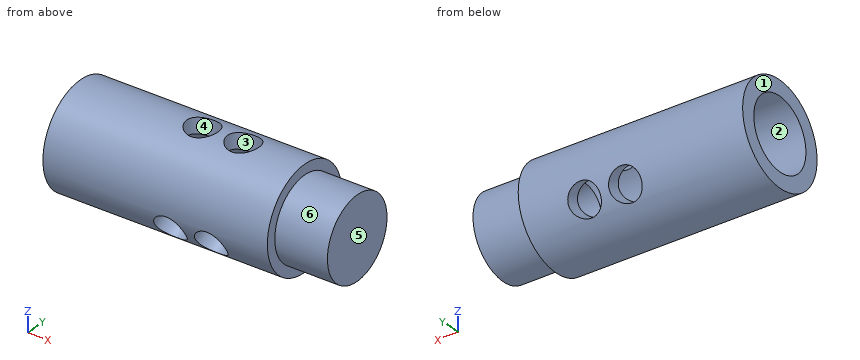
Autodesk Inventor part; units mm, degrees
ref_plane "YZ Plane" through (0, 0, 0) normal (1, 0, 0) x (0, 1, 0)
ref_plane "XZ Plane" through (0, 0, 0) normal (0, 1, 0) x (-1, 0, 0)
ref_plane "XY Plane" through (0, 0, 0) normal (0, 0, 1) x (1, 0, 0)
sketch "Sketch4" plane through (0, 0, 0) normal (0, 0, 1) x (1, 0, 0)
  line L0 (0, 0) -> (0, 5.5562) construction
  line L1 (0, 5.5562) -> (20.1197, 5.5563)
  line L2 (0, 7.9375) -> (26.1937, 7.9375)
  line L3 (26.1937, 7.9375) -> (26.1937, 6.35)
  line L4 (26.1937, 5.5563) -> (26.1937, 0) construction
  line L5 (26.1937, 0) -> (0, 0) construction
  line L6 (26.1937, 6.35) -> (34.3852, 6.35)
  line L7 (26.1937, 0) -> (31.75, 0) construction
  line L8 (34.3852, 0) -> (34.3852, 6.35)
  line L9 (16.6687, 7.9375) -> (16.6687, 0) construction
  circle A0 centre (16.6687, 7.5565) radius 2.3813 construction
  circle A1 centre (16.6687, 5.4928) radius 2.3813 construction
  circle A2 centre (10.3187, 7.5565) radius 2.3813 construction
  circle A3 centre (10.3187, 5.4928) radius 2.3813 construction
  line L10 (10.3187, 7.9375) -> (10.3187, 0) construction
  line L11 (0, 5.1753) -> (26.1938, 5.1753) construction
  line L12 (8.7312, 5.1753) -> (8.7312, 0) construction
  line L13 (5.5562, 5.1753) -> (5.5562, 0) construction
  line L14 (18.2563, 5.1753) -> (18.2562, 0) construction
  line L15 (21.4313, 5.1753) -> (21.4312, 0) construction
  line L16 (0, 3.1115) -> (26.1937, 3.1115) construction
  line L17 (5.5562, 3.1115) -> (8.7312, 5.1753) construction
  line L18 (18.2563, 5.1753) -> (21.4312, 3.1115) construction
  line L19 (11.9062, 5.1753) -> (11.9062, 0) construction
  line L20 (15.0812, 5.1753) -> (15.0812, 0) construction
  line L21 (11.9062, 5.1753) -> (15.0812, 3.1115) construction
  line L22 (21.4312, 3.3734) -> (29.723, 3.3734)
  line L23 (24.6062, 3.3734) -> (24.6062, 0) construction
  line L24 (21.4312, 3.3734) -> (20.1197, 5.5563)
  line L25 (26.1937, 3.1115) -> (30.9562, 3.1115) construction
  line L26 (30.9562, 3.1115) -> (30.9562, 0) construction
  line L27 (31.75, 3.3734) -> (31.75, 0) construction
  line L28 (31.75, 0) -> (29.723, 3.3734)
  line L29 (0, 7.9375) -> (-1.5875, 7.9375) construction
  line L30 (-1.5875, 7.9375) -> (-1.5875, 3.3734) construction
  line L31 (-1.5875, 3.3734) -> (5.5562, 3.3734) construction
  line L32 (0, 5.5562) -> (0, 7.9375)
  line L33 (0, 7.9375) -> (0, 12.7) construction
  line L34 (20.1197, 5.5563) -> (26.1937, 5.5563) construction
  line L35 (29.723, 3.3734) -> (34.3852, 3.3734) construction
  line L36 (26.1937, 6.35) -> (26.1937, 5.5563) construction
  line L37 (31.75, 0) -> (34.3852, 0)
  line L38 (0, 5.5562) -> (-8.7313, 5.5563)
  line L39 (-8.7313, 5.5563) -> (-8.7313, 7.9375)
  line L40 (-8.7313, 7.9375) -> (0, 7.9375)
  line L41 (-8.7313, 6.35) -> (0, 6.35)
  dimension "d16" = 12.7
  dimension "d17" = 5.5563
  dimension "d18" = 7.9375
  dimension "d19" = 26.1938
  dimension "d20" = 8.1915
  dimension "d21" = 6.35
  dimension "d22" = 9.525
  dimension "d23" = 6.35
  dimension "d24" = 0.381
  dimension "d25" = 0.381
  dimension "d26" = 0.0635
  dimension "d27" = 0.0635
  dimension "d28" = 1.5875
  dimension "d29" = 4.7625
  dimension "d30" = 1.5875
  dimension "d31" = 4.7625
  dimension "d32" = 3.1115
  dimension "d33" = 1.5875
  dimension "d34" = 4.7625
  dimension "d35" = 3.3734
  dimension "d36" = 3.175
  dimension "d37" = 31
  dimension "d38" = 9.525
  dimension "d39" = 9.525
  dimension "d40" = 0.7937
  dimension "d41" = 31
  dimension "d42" = 1.5875
  dimension "d43" = 3.3734
  dimension "d49" = 4.7625
  dimension "d63" = 8.7312
  dimension "d64" = 6.35
revolve "Revolution1" add sketch "Sketch4" angle 360 about axis through (26.1937, 0, 0) along (-1, 0, 0)
sketch "Sketch5" plane through (0, 0, 0) normal (0, 0, 1) x (1, 0, 0)
  line L0 (26.1937, -7.9375) -> (26.1937, 7.9375)
  line L1 (0, 0) -> (26.1937, 0) construction
  circle A0 centre (16.6687, 0) radius 2.4574
  circle A1 centre (10.3187, 0) radius 2.4574
  dimension "d51" = 4.9149
  dimension "d53" = 6.35
  dimension "d54" = 9.525
  dimension "d55" = 4.9149
extrude "Extrusion4" cut sketch "Sketch5" along normal through all
pattern_circular "Circular Pattern2" count 3 over 360 about axis through (-4.3656, 0, 0) along (1, 0, 0) of "Extrusion4"
ref_plane "Work Plane1" through (16.6687, 0, 0) normal (1, 0, 0) x (0, 0, -1)
ref_plane "Work Plane2" through (10.3187, 0, 0) normal (1, 0, 0) x (0, 0, -1)
equation "\"d17\" = d44"
equation "\"d18\" = d45"
equation "\"d24\" = d46"
equation "\"d25\" = d24"
equation "\"d26\" = d47"
equation "\"d27\" = d26"
equation "\"d32\" = d48"
equation "\"d33\" = d28"
equation "\"d34\" = d29"
equation "\"d39\" = d38"
equation "\"d41\" = d37"
equation "\"d43\" = d35"
equation "\"d55\" = d51"
properties part number "Output SHaft"
Can you work these out from the model? Positions are in its coordinate system, mm. Face numbers are marked on the shaded views. A direction names the side the tool comes from. Round coordinates to 2 decimals unless told otherwise and drop trailing zeros. Loops run counter-clockwise (first coordinate to the right, second up) from the corner with the lowest first, then second, coordinate; pieces in that order, holes last. Notation, with made-up numbers: M 4.25,-31 L 23.25,-31 A26 ccw 23.25,-8 Z; hole C 50.5,-10.5 d2. An arc over 180 degrees is marked long. Answer as a JSON object with one key per item and string values. Group by question number.
Q1. On a 3-axis mill with a long thin cutter (end or side, diameter ignored), from which of +Z, -Z, +X, -X, +Y, -Y can I reach the whole of each face in a straight line? I mean the marked faces 1, 2 and 3. Say none if no direction works.
Q2. Imagine slicing it at A-A, the plane x = 28. Please give me the cut outline in (y, z), then the cut area to 3 significant figures.
Q3. Imagine slicing it at B-B, the plane x = 11.5. Please give me the cut outline in (y, z) (1 decimal), then the cut area to 3 significant figures.
Q4. Will these pins go through, and if not, where does the flat tip stop? pin 1 (3 mm diameter, centred on x = 27.5, z = -4.5, fed in from +Y); pin 2 (1.5 mm diameter, centred on x = 25.5, y = -1, fed in from +Z); pin 3 (3 mm diameter, centred on x = 16.67, y = 0, fed in from +Z).
Q5. Imagine slicing it at C-C, the plane x = 5. Please give me the cut outline in (y, z) (1 decimal), then the cut area to 3 significant figures.
Q6. We'd pull the mould along Y, two halves only. Please class the marked faces 4, 5 and 6: +Y half, -Y half, draft (parallel to the pull), parting line (faces both ways), or undercut.
Q7. Please list where these lines run through material, in increasing order: L1, parallel to Y at x = 13, z = 0; L2, parallel to X at y = 0, z = 6.
Findings:
{
 "1": {"face 1": "+Z, -Z, -X, +Y, -Y", "face 2": "-X", "face 3": "+Z"},
 "2": {"outline": "C 0,0 d12.7; hole C 0,0 d6.75", "area": "90.9 mm2"},
 "3": {"outline": "M -7.7,-2 L -5.5,-0.7 A5.6 cw -2.2,5.1 L -2.2,7.6 A7.9 ccw Z; M -5.5,-5.7 A7.9 ccw 5.5,-5.7 L 3.4,-4.4 A5.6 cw -3.4,-4.4 Z; M 2.2,5.1 A5.6 cw 5.5,-0.7 L 7.7,-2 A7.9 ccw 2.2,7.6 Z", "area": "69.6 mm2"},
 "4": {"pin 1": "stops at y = 6.99", "pin 2": "stops at z = 7.93", "pin 3": "stops at z = -5.35"},
 "5": {"outline": "C 0,0 d15.9; hole C 0,0 d11.1", "area": "101 mm2"},
 "6": {"face 4": "undercut", "face 5": "draft", "face 6": "parting line"},
 "7": {"L1": "y = -7.94 to -5.56, 5.56 to 7.94", "L2": "x = -8.73 to 7.86, 12.78 to 14.21, 19.13 to 34.39"}
}
